Read the model definition and answer for the solid it produces. Units are mm, in the model's axes. Give positions to 0.01 mm unless a question says otherwise; leave off trailing zeros. Write each loop counter-clockwise with the first axis right and the second up, starting at its lowest first coordinate (ties: lowest second). Pieces come first, ordered by that corner, then holes. Notation, with made-up numbers: M 33.5,15 L 41.5,15 A29 ccw 41.5,51 Z; hole C 10,68.5 d10. An arc over 180 degrees is marked long. Put each result on its own line as item: value.
from build123d import *

# Parameters (mm, degrees)
F1_DEPTH = 6.35


with BuildPart() as f1:
    # F0 (on Top) → F1 (new body)
    with BuildSketch(Plane.XY):
        Polygon((538.830596, 268.757908), (339.87359, -75.845721), (374.275071, -135.430819), (772.189058, -135.430819), (806.590538, -75.845721), (607.633532, 268.757908), align=None)
        with BuildLine():
            ThreePointArc((396.296871, -126.878334), (399.675071, -123.500134), (403.053271, -126.878334))
            ThreePointArc((403.053271, -126.878334), (399.675071, -130.256534), (396.296871, -126.878334))
        make_face(mode=Mode.SUBTRACT)
        with BuildLine():
            ThreePointArc((356.602055, -58.124903), (359.980255, -54.746703), (363.358455, -58.124903))
            ThreePointArc((363.358455, -58.124903), (359.980255, -61.503103), (356.602055, -58.124903))
        make_face(mode=Mode.SUBTRACT)
        with BuildLine():
            ThreePointArc((569.853877, -126.878334), (573.232077, -123.500134), (576.610277, -126.878334))
            ThreePointArc((576.610277, -126.878334), (573.232077, -130.256534), (569.853877, -126.878334))
        make_face(mode=Mode.SUBTRACT)
        with BuildLine():
            ThreePointArc((743.410858, -126.878334), (746.789058, -123.500134), (750.167258, -126.878334))
            ThreePointArc((750.167258, -126.878334), (746.789058, -130.256534), (743.410858, -126.878334))
        make_face(mode=Mode.SUBTRACT)
        with BuildLine():
            ThreePointArc((783.105673, -58.124903), (786.483873, -54.746703), (789.862073, -58.124903))
            ThreePointArc((789.862073, -58.124903), (786.483873, -61.503103), (783.105673, -58.124903))
        make_face(mode=Mode.SUBTRACT)
        with BuildLine():
            ThreePointArc((443.380571, 92.179851), (446.758771, 95.558051), (450.136971, 92.179851))
            ThreePointArc((450.136971, 92.179851), (446.758771, 88.801651), (443.380571, 92.179851))
        make_face(mode=Mode.SUBTRACT)
        with BuildLine():
            ThreePointArc((696.327157, 92.179851), (699.705357, 95.558051), (703.083557, 92.179851))
            ThreePointArc((703.083557, 92.179851), (699.705357, 88.801651), (696.327157, 92.179851))
        make_face(mode=Mode.SUBTRACT)
        with BuildLine():
            ThreePointArc((530.159062, 242.484631), (533.537262, 245.862831), (536.915462, 242.484631))
            ThreePointArc((536.915462, 242.484631), (533.537262, 239.106431), (530.159062, 242.484631))
        make_face(mode=Mode.SUBTRACT)
        with BuildLine():
            ThreePointArc((609.548667, 242.484631), (612.926867, 245.862831), (616.305067, 242.484631))
            ThreePointArc((616.305067, 242.484631), (612.926867, 239.106431), (609.548667, 242.484631))
        make_face(mode=Mode.SUBTRACT)
    extrude(amount=F1_DEPTH)


solid = f1.part
(1) Given pin 1 Ø3 at (x, y) = (594, 178) entering from -Z; pin 2 Ø5 at (x, y) = (666, 173.5) entering from +Z, each flat-ended and moving along its own axis, determine where each tip first touches the part or whether it passes through.
Result:
pin 1: stops at z = 0
pin 2: passes through
(2) Section B-B on y = 163 is taken. Determine the outline of the cut face in (x, z).
Result:
outline: M 477.77,0 L 668.69,0 L 668.69,6.35 L 477.77,6.35 Z
(3) Straight lines are drawn through the part: line 1 along Y through (x, z) = (785, 4.5); line 2 along Y through (x, z) = (526.5, 1.5); line 3 along Y through (x, z) = (632, 2). For each, find the intervals that lie inside material, in ascending order. Write a range as from..to.
Result:
line 1: y = -113.24..-61.16, -55.09..-38.45
line 2: y = -135.43..247.4
line 3: y = -135.43..226.55
(4) Section A-A on z = 3.25 is taken. Give the number of separate pieces and of enclosed holes in the cut face, and give its area (3 significant figures).
Result:
separate pieces: 1
enclosed holes: 9
area: 118,000 mm²
(5) Section C-C on x = 637.5 is taken. Determine the outline of the cut face in (y, z).
Result:
outline: M -135.43,0 L 217.03,0 L 217.03,6.35 L -135.43,6.35 Z
